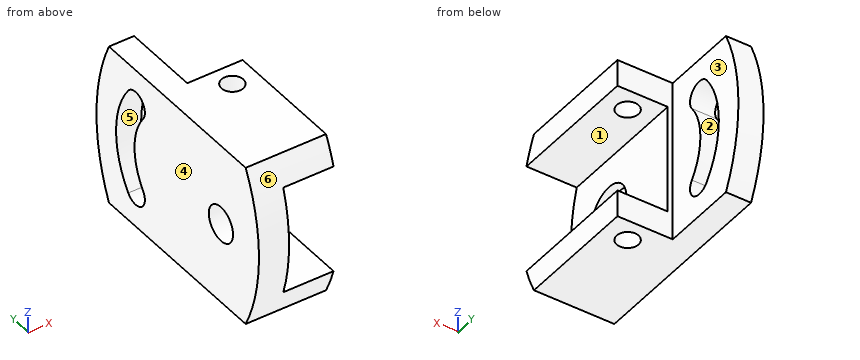
Autodesk Inventor part; units mm, degrees
ref_plane "YZ Plane" through (0, 0, 0) normal (1, 0, 0) x (0, 1, 0)
ref_plane "XZ Plane" through (0, 0, 0) normal (0, 1, 0) x (-1, 0, 0)
ref_plane "XY Plane" through (0, 0, 0) normal (0, 0, 1) x (1, 0, 0)
sketch "Sketch1" plane through (0, 0, 0) normal (1, 0, 0) x (0, 1, 0)
  arc A0 (11.5026, 48.5) -> (11.5026, -48.5) centre (108, 0) ccw
  arc A1 (130.1868, -48.5) -> (130.1868, 48.5) centre (26.826, 0) ccw
  line L0 (11.5026, 48.5) -> (130.1868, 48.5)
  line L1 (130.1868, -48.5) -> (11.5026, -48.5)
  line L2 (0, 0) -> (141, 0)
  arc A2 (107, -27) -> (107, 27) centre (71, 0) ccw construction
  arc A3 (113.4, -31.8) -> (113.4, 31.8) centre (71, 0) ccw
  arc A4 (100.6, -22.2) -> (100.6, 22.2) centre (71, 0) ccw
  arc A5 (100.6, -22.2) -> (113.4, -31.8) centre (107, -27) ccw
  arc A6 (113.4, 31.8) -> (100.6, 22.2) centre (107, 27) ccw
  dimension "d0" = 108
  dimension "d2" = 141
  dimension "d3" = 97
  dimension "d4" = 54
  dimension "d5" = 8
  dimension "d6" = 45
extrude "Extrusion1" add sketch "Sketch1" along normal blind 48 contours L0 A1 L2 A3 A6 A4 A0 | L2 A4 A5 A3 A1 L1 A0
sketch "Sketch2" plane through (48, 0, 0) normal (1, 0, 0) x (0, 0, -1)
  line L0 (-88.6528, 151.7053) -> (89.775, 151.7053)
  line L1 (89.775, 151.7053) -> (89.775, 84)
  line L2 (89.775, 84) -> (-88.6528, 84)
  line L3 (-88.6528, 84) -> (-88.6528, 151.7053)
  point P0 (0, 0)
  dimension "d9" = 84
extrude "Extrusion2" cut sketch "Sketch2" against normal blind 33
sketch "Sketch3" plane through (48, 0, 0) normal (1, 0, 0) x (0, 0, -1)
  line L0 (48.5, 84) -> (-48.5, 84)
  line L1 (-32.5, 84) -> (32.5, 84)
  line L2 (32.5, 84) -> (32.5, -13.4662)
  line L3 (32.5, -13.4662) -> (-32.5, -13.4662)
  line L4 (-32.5, -13.4662) -> (-32.5, 84)
  line L5 (-48.5, 84) -> (-48.5, 11.5026)
  line L6 (48.5, 11.5026) -> (48.5, 84)
  point P0 (0, 0)
  dimension "d12" = 16
  dimension "d13" = 16
extrude "Extrusion3" cut sketch "Sketch3" against normal blind 30
sketch "Sketch4" plane through (0, 11.5026, 48.5) normal (0, 0, 1) x (1, 0, 0)
  circle A0 centre (33, 59.4974) radius 6.5
  line L0 (48, 72.4974) -> (15, 72.4974)
  line L1 (48, 72.4974) -> (48, 0)
  point P0 (0, -11.5026)
  dimension "d16" = 13
  dimension "d17" = 13
  dimension "d18" = 15
extrude "Extrusion4" cut sketch "Sketch4" against normal through all
sketch "Sketch5" plane through (18, 0, 0) normal (1, 0, 0) x (0, 0, -1)
  point P0 (0, 0)
  point P1 (0, 33)
  dimension "d21" = 33
hole "Hole1" at (18, 33, 0) direction (-1, 0, 0) diameter 21 end through all counterbore diameter 30 counterbore depth 6
properties part number "swivel plate"
CAD build for the part. Positions are in the model's coordinates, mm. Face numbers are marked on the shaded views. A direction names the side the tool comes from. Round coordinates to 2 decimals unless told otherwise and drop trailing zeros. Write each loop counter-clockwise with the first axis right and the second up, starting at its lowest first coordinate (ties: lowest second). Pieces come first, ordered by that corner, then holes. Notation, with made-up numbers: M -33.5,64 L -16.5,64 A16 ccw -16.5,70 Z; hole C 48,36 d11. An arc over 180 degrees is marked long. Use a Markdown table: item, result. Add a question column.
1. Flat gauge pins, fed straight in: P1, Ø5, axis at x = 8, z = -38.5, coming from the -Y side; P2, Ø10.5, axis at x = 33, y = 71, coming from the -Z side; P3, Ø10, axis at y = 75.5, z = 3.5, coming from the +X side; P4, Ø12, axis at y = 119.5, z = -31, coming from the +X side. Where does each tip first touch, or does it go through?
2. Slice it at D-D on x = 6. Give the cut face in (y, z), then the cut area to 3 significant figures.
3. Drill centre lines: probe 1 along Z at (x, y) = (40.5, 82.5); probe 2 along Z at (x, y) = (16.55, 33); probe 3 along X at (y, z) = (12, -11.5). Where is each one in solid material? Low to high.
4. Slice it at A-A on y = 33. Give the cut face in (x, z), then the cut area to 3 significant figures.
5. Pull direction Z, two halves, no side cores. Call the marked faces 4, 5 and 6: released by +Z, released by -Z, zero draft, split by the parting line, or undercut.
6. Slice it at C-C on z = 0. Give the cut face in (x, y).
7. Slice it at B-B on x = 33. Give the cut face in (y, z).
8. 3-axis set-ups, long thin cutter, end or side, ignore diameter. For the marked faces 1, 2 and 3: which of +Z, -Z, +X, -X, +Y, -Y reach the whole face in a straight line?
Reply:
| question | item | result |
|---|---|---|
| 1 | P1 | stops at y = 6.18 |
| 1 | P2 | passes through |
| 1 | P3 | stops at x = 18 |
| 1 | P4 | stops at x = 15 |
| 2 | outline | M 11.5,-48.5 L 130.19,-48.5 A114.17 ccw 130.19,48.5 L 11.5,48.5 A108 ccw Z; hole C 33,0 d21; hole M 100.6,-22.2 A8 ccw 113.4,-31.8 A53 ccw 113.4,31.8 A8 ccw 100.6,22.2 A37 cw Z |
| 2 | area | 11,500 mm^2 |
| 3 | probe 1 | z = -48.5 to -32.5, 32.5 to 48.5 |
| 3 | probe 2 | z = -48.5 to -15, 15 to 48.5 |
| 3 | probe 3 | x = 0 to 18 |
| 4 | outline | M 0,-48.5 L 48,-48.5 L 48,-32.5 L 18,-32.5 L 18,-15 L 12,-15 L 12,-10.5 L 0,-10.5 Z; M 0,10.5 L 12,10.5 L 12,15 L 18,15 L 18,32.5 L 48,32.5 L 48,48.5 L 0,48.5 Z |
| 4 | area | 2,270 mm^2 |
| 5 | face 4 | zero draft |
| 5 | face 5 | undercut |
| 5 | face 6 | split by the parting line |
| 6 | outline | M 0,0 L 18,0 L 18,18 L 12,18 L 12,22.5 L 0,22.5 Z; M 0,43.5 L 12,43.5 L 12,48 L 18,48 L 18,84 L 15,84 L 15,108 L 0,108 Z; M 0,124 L 15,124 L 15,141 L 0,141 Z |
| 7 | outline | M 5.01,-32.5 A108 ccw 11.5,-48.5 L 64.5,-48.5 L 64.5,-32.5 Z; M 5.01,32.5 L 64.5,32.5 L 64.5,48.5 L 11.5,48.5 A108 ccw Z; M 77.5,-48.5 L 84,-48.5 L 84,-32.5 L 77.5,-32.5 Z; M 77.5,32.5 L 84,32.5 L 84,48.5 L 77.5,48.5 Z |
| 8 | face 1 | +X, +Y, -Y |
| 8 | face 2 | +X, -X |
| 8 | face 3 | +Z, -Z, +X, +Y |
